Autodesk Fusion 360 part; units mm, degrees
box "BoxPrimitive1" add length 8 width 28 height 14 placed x (0, 0, 1) y (1, 0, 0) z (0, 1, 0) at (-28, 0, 0)
box "BoxPrimitive2" add length 8 width 15 height 20 placed x (0, 0, 1) y (1, 0, 0) z (0, 1, 0) at (-15, 14, 0)
sketch "Sketch4" plane through (0, 0, 8) normal (0, 0, 1) x (1, 0, 0)
  line L0 (-28, 14) -> (-28, 0)
  line L1 (-28, 0) -> (0, 0)
  line L2 (0, 0) -> (0, 34)
  line L3 (0, 34) -> (-15, 34)
  line L4 (-15, 34) -> (-15, 14)
  line L5 (-15, 14) -> (-28, 14)
  line L6 (-15, 34) -> (0, 34)
  line L7 (0, 34) -> (0, 14)
  line L8 (0, 14) -> (-15, 14)
  line L9 (-15, 14) -> (-15, 34)
  line L10 (-7.5, 34) -> (-7.5, 14) construction
  point P0 (-7.5, 27)
  dimension "holeHeight" = 13
hole "Hole1" at (-7.5, 27, 8) direction (0, 0, -1) diameter 8.5 end through all
extrude "Extrude1" cut sketch "Sketch4" against normal blind 1.5 contours L2 L3 L4 L6 L7 L8 L9
fillet "Fillet2" radius 7 2 edges at (-15, 34, 3.25) (0, 34, 3.25)
fillet "Fillet3" radius 4 1 edges at (-15, 14, 3.25)
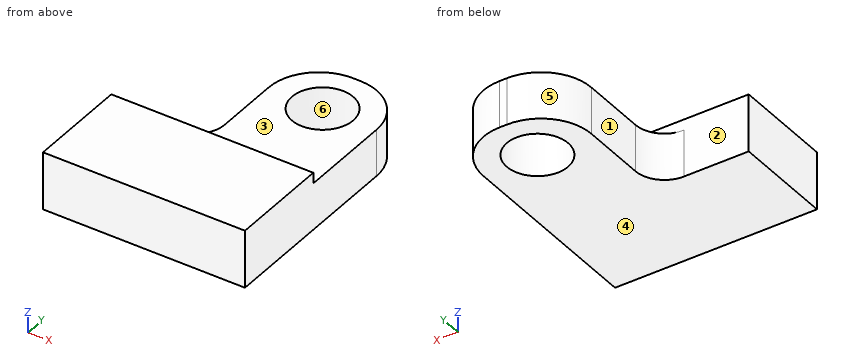
The model under review builds one solid part; all positions refer to its coordinate system, in mm. Face numbers are marked on the shaded views. A direction names the side the tool comes from. Coordinates: 2 decimals unless noted, no trailing zeros. Write each loop counter-clockwise with the first axis right and the second up, starting at its lowest first coordinate (ties: lowest second). Pieces come first, ordered by that corner, then holes. Notation, with made-up numbers: (2, 60) - (38, 60) arc R21 cw to (38, 87) - close; hole circle Ø5 at (60.5, 81). An arc over 180 degrees is marked (long way). Answer as a JSON object with one key per item and string values. Group by question number.
1. Mouldability with a two-part tool opening along Y and no side actions: class the marked faces 4, 5 and 6 as pulls with the +Y half, pulls with the -Y half, needs draft (parallel to the pull), parting line crosses it, or undercut.
2. Add section A-A (x = -7.5). Give the boundary of the cut face in (y, z), plus the area to 3 significant figures.
3. Add section B-B (z = 2). Give the boundary of the cut face in (x, y).
4. Add section D-D (x = -12.25). Give the boundary of the cut face in (y, z), plus the area to 3 significant figures.
5. Machinability: for the marked faces 1, 2 and 3, which of the approach directions +Z, -Z, +X, -X, +Y, -Y give a long, thin tool a straight path to every point of the face, cutting with its end or side? Answer none if there is none.
6. To check wall thickness, follow probe 1 along X at (y, z) = (27, 3); probe 2 along Y at (x, z) = (-7.5, 3.5); probe 3 along X at (y, z) = (21, 5.25). State the ranges of each line that lie inside material, in increasing order.
7. Add section C-C (x = -4.5). Give the boundary of the cut face in (y, z).
8. Clearance check with flat-ended pins moving along their axes: pin 1 Ø1.5 at (y, z) = (17.5, 2.5) entering from -X; pin 2 Ø2 at (x, y) = (-5, 29) entering from +Z; pin 3 Ø3 at (y, z) = (23.5, 2) entering from -X; pin 4 Ø15 at (x, y) = (-12, 22.5) entering from +Z. State where each tip first meets the part, or that it passes through.
Findings:
{
 "1": {"face 4": "needs draft", "face 5": "pulls with the +Y half", "face 6": "undercut"},
 "2": {"outline": "(0, 0) - (22.75, 0) - (22.75, 6.5) - (14, 6.5) - (14, 8) - (0, 8) - close; (31.25, 0) - (34, 0) - (34, 6.5) - (31.25, 6.5) - close", "area": "187 mm²"},
 "3": {"outline": "(-28, 0) - (0, 0) - (0, 27) arc R7 ccw to (-7, 34) - (-8, 34) arc R7 ccw to (-15, 27) - (-15, 18) arc R4 cw to (-19, 14) - (-28, 14) - close; hole circle Ø8.5 at (-7.5, 27)"},
 "4": {"outline": "(0, 0) - (32.56, 0) - (32.56, 6.5) - (14, 6.5) - (14, 8) - (0, 8) - close", "area": "233 mm²"},
 "5": {"face 1": "+Z, -Z, -X, +Y", "face 2": "+Z, -X, +Y", "face 3": "+Z, +X, -X, +Y"},
 "6": {"probe 1": "-15 to -11.75, -3.25 to 0", "probe 2": "0 to 22.75, 31.25 to 34", "probe 3": "-15 to 0"},
 "7": {"outline": "(0, 0) - (23.99, 0) - (23.99, 6.5) - (14, 6.5) - (14, 8) - (0, 8) - close; (30.01, 0) - (33.54, 0) - (33.54, 6.5) - (30.01, 6.5) - close"},
 "8": {"pin 1": "x = -15.2", "pin 2": "through", "pin 3": "x = -15", "pin 4": "z = 6.5"}
}
